Work out the finished part from the listing and answer in its coordinate system (mm). Face numbers are marked on the shaded views. A direction names the side the tool comes from. Round coordinates to 2 decimals unless told otherwise and drop trailing zeros. Order: outer loops, then holes, each group sorted by start corner. A loop starts at its lowest first (then second) coordinate and runs counter-clockwise, first axis right, second up. Notation, with made-up numbers: (7, -7) -> (53, -7) arc R28 ccw to (53, 24) -> close; hole circle Ø4 at (-23, -31). An arc over 180 degrees is marked (long way). Use a Markdown table: item, result. Add a question column.
Item 1: A cutting plane is placed at C-C, the plane y = -2. Determine the outline of the cut face in (x, z).
Item 2: A cutting plane is placed at A-A, the plane z = 31. Determine the outline of the cut face in (x, y).
Item 3: Find the intervals of material crossed by L1, parallel to Y at x = 39, z = -0.5; L2, parallel to Z at x = 40, y = 28; L3, parallel to Z at x = 20, y = -25.5, in increasing order. Write a range as [from, to].
Item 4: For a pull along Y with two mould halves and no side action, classify the marked faces 4, 5, 6 and 7 as +Y half, -Y half, draft (parallel to the pull), parting line (faces both ways), or undercut.
Item 5: A cutting plane is placed at D-D, the plane z = 9.5. Determine the outline of the cut face in (x, y), plus the area to 3 significant figures.
Item 6: A tool of negligible diameter and unlimited length cuts with its end or side. For the marked faces 1, 2 and 3, from which of +Z, -Z, +X, -X, +Y, -Y can it reach the whole face along a straight path? Write none if from no direction.
Item 7: Flat-ended cylindrical pins translate along their axes: P1, Ø1, axis at x = 70.5, z = 5, coming from the +Y side; P2, Ø1.5, axis at x = 111.5, z = 25, coming from the +Y side; P3, Ø10, axis at x = 97, z = 13.5, coming from the +Y side. Find the tip coordinate at first contact, or state that the pin passes through.
from build123d import *

# Parameters (mm, degrees)
F0_R     = 38.1
F1_DEPTH = 203.2
F3_DEPTH = 228.6


with BuildPart() as f1:
    # F0 (on Right) → F1 (new body)
    with BuildSketch(Plane.YZ):
        Circle(F0_R)
    extrude(amount=F1_DEPTH)

    # F2 (on face) → F3 (cut)
    with BuildSketch(Plane.YZ.offset(203.2)):
        with BuildLine():
            Line((12.7, 35.9210244843), (12.7, 25.4))
            Line((12.7, 25.4), (28.3980633142, 25.4))
            ThreePointArc((28.3980633142, 25.4), (21.211687606, 31.6492386781), (12.7, 35.9210244843))
        make_face()
        with BuildLine():
            ThreePointArc((37.9042612368, 3.8570688473), (35.7635714939, 13.1368547986), (31.3883642677, 21.595846559))
            Line((31.3883642677, 21.595846559), (25.2042612368, 13.084158953))
            Line((25.2042612368, 13.084158953), (37.9042612368, 3.8570688473))
        make_face()
        with BuildLine():
            ThreePointArc((32.9323196853, -19.1591315081), (36.6549866302, -10.3933611087), (38.0874402363, -0.9782107359))
            Line((38.0874402363, -0.9782107359), (28.0813513425, -4.2293860998))
            Line((28.0813513425, -4.2293860998), (32.9323196853, -19.1591315081))
        make_face()
        with BuildLine():
            ThreePointArc((15.3813513425, -34.8571948223), (23.545442731, -29.9536663299), (30.2384085792, -23.1786247779))
            Line((30.2384085792, -23.1786247779), (20.2323196853, -19.9274494141))
            Line((20.2323196853, -19.9274494141), (15.3813513425, -34.8571948223))
        make_face()
        with BuildLine():
            Line((-4.6552295797, 28.0139043612), (8.0447704203, 37.2409944669))
            ThreePointArc((8.0447704203, 37.2409944669), (-1.4423399886, 38.0726891007), (-10.8393326105, 36.5255919673))
            Line((-10.8393326105, 36.5255919673), (-4.6552295797, 28.0139043612))
        make_face()
        with BuildLine():
            Line((-25.2042612368, -13.084158953), (-37.9042612368, -3.8570688473))
            ThreePointArc((-37.9042612368, -3.8570688473), (-35.7635714939, -13.1368547986), (-31.3883642677, -21.595846559))
            Line((-31.3883642677, -21.595846559), (-25.2042612368, -13.084158953))
        make_face()
        with BuildLine():
            Line((-12.7, -25.4), (-28.3980633142, -25.4))
            ThreePointArc((-28.3980633142, -25.4), (-21.211687606, -31.6492386781), (-12.7, -35.9210244843))
            Line((-12.7, -35.9210244843), (-12.7, -25.4))
        make_face()
        with BuildLine():
            ThreePointArc((-8.0447704203, -37.2409944669), (1.4423399886, -38.0726891007), (10.8393326105, -36.5255919673))
            Line((10.8393326105, -36.5255919673), (4.6552295797, -28.0139043612))
            Line((4.6552295797, -28.0139043612), (-8.0447704203, -37.2409944669))
        make_face()
        with BuildLine():
            Line((-28.0813513425, 4.2293860998), (-32.9323196853, 19.1591315081))
            ThreePointArc((-32.9323196853, 19.1591315081), (-36.6549866302, 10.3933611087), (-38.0874402363, 0.9782107359))
            Line((-38.0874402363, 0.9782107359), (-28.0813513425, 4.2293860998))
        make_face()
        with BuildLine():
            Line((-20.2323196853, 19.9274494141), (-15.3813513425, 34.8571948223))
            ThreePointArc((-15.3813513425, 34.8571948223), (-23.545442731, 29.9536663299), (-30.2384085792, 23.1786247779))
            Line((-30.2384085792, 23.1786247779), (-20.2323196853, 19.9274494141))
        make_face()
    extrude(amount=-F3_DEPTH, mode=Mode.SUBTRACT)


solid = f1.part
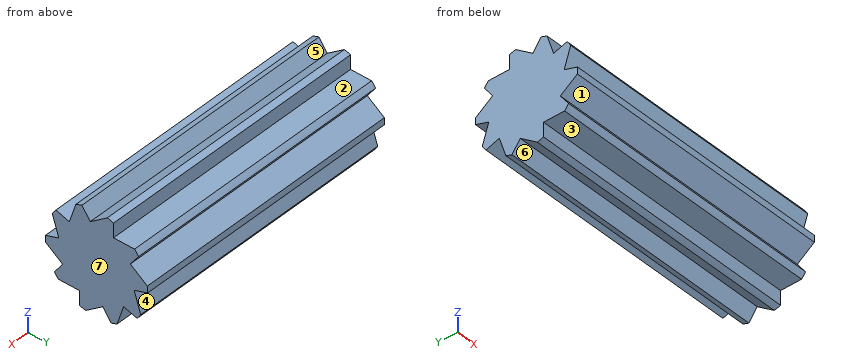
Reported:
| question | item | result |
|---|---|---|
| 1 | outline | (0, -32.85) -> (203.2, -32.85) -> (203.2, 29.94) -> (0, 29.94) -> close |
| 2 | outline | (0, -16.63) -> (203.2, -16.63) -> (203.2, -6.82) -> (0, -6.82) -> close; (0, -0.55) -> (203.2, -0.55) -> (203.2, 12.7) -> (0, 12.7) -> close |
| 3 | L1 | [-38.1, 38.1] |
| 3 | L2 | [-22.45, 11.05], [16.93, 25.4] |
| 3 | L3 | [-25.4, -13.49], [-12.87, 21.64] |
| 4 | face 4 | +Y half |
| 4 | face 5 | undercut |
| 4 | face 6 | undercut |
| 4 | face 7 | draft |
| 5 | outline | (0, -29.79) -> (203.2, -29.79) -> (203.2, 30.14) -> (0, 30.14) -> close |
| 5 | area | 12,200 mm² |
| 6 | face 1 | +X, -X, -Y |
| 6 | face 2 | +Z, +X, -X, +Y |
| 6 | face 3 | -Z, +X, -X, -Y |
| 7 | P1 | y = 37.02 |
| 7 | P2 | y = 29.39 |
| 7 | P3 | y = 31.51 |
